```python
from build123d import *

# Parameters (mm, degrees)
BOSS_EXTRUDE1_DEPTH      = 4.5
BOSS_EXTRUDE1_DEPTH_BACK = 4.5
SKETCH1_R                = 11.1125
SKETCH1_R_2              = 4.7625
FILLET1_R                = 1
FILLET2_R                = 1


with BuildPart() as part:
    # Sketch1 → Boss-Extrude1 (new, two sides: drawn at the far end of the back side and taken through both)
    with BuildSketch(Plane(origin=(0, 0, 0), x_dir=(1, 0, 0), z_dir=(0, 1, 0)).offset(-BOSS_EXTRUDE1_DEPTH_BACK)):
        with Locations(Location((0, 0, 0), (0, 0, 270))):
            Circle(SKETCH1_R)
        with Locations(Location((0, 0, 0), (0, 0, 270))):
            Circle(SKETCH1_R_2, mode=Mode.SUBTRACT)
    extrude(amount=BOSS_EXTRUDE1_DEPTH + BOSS_EXTRUDE1_DEPTH_BACK)

    # Fillet1
    fillet1_edges = [part.edges().sort_by_distance(p)[0] for p in [
        (0, -4.5, -4.7625),
        (0, 4.5, -4.7625),
    ]]
    fillet(fillet1_edges, radius=FILLET1_R)

    # Fillet2
    fillet2_edges = [part.edges().sort_by_distance(p)[0] for p in [
        (0, -4.5, -11.1125),
        (0, 4.5, -11.1125),
    ]]
    fillet(fillet2_edges, radius=FILLET2_R)


solid = part.part
```
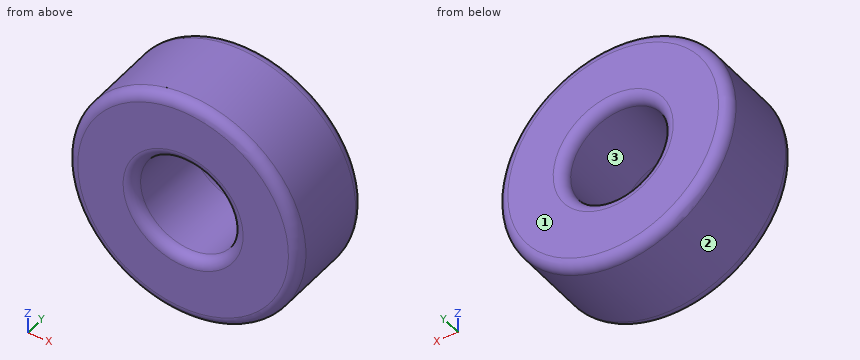
For this review, take the finished solid that the model builds, in its own axes (mm). Face numbers are marked on the shaded views. Give positions to 0.01 mm unless a question says otherwise; leave off trailing zeros. Order: outer loops, then holes, each group sorted by start corner. A loop starts at its lowest first (then second) coordinate and runs counter-clockwise, first axis right, second up.
1) Take a section at B-B (z = 0). Give the boundary of the cut face in (x, y), then the cut area to 3 significant figures.
2) Take a section at A-A (x = 0). Give the boundary of the cut face in (y, z).
3) Take a section at C-C (y = -2.75). Give the boundary of the cut face in (x, z) (1 decimal), then the cut area to 3 significant figures.
4) Wall thickness on line 1 (X direction, y = -2, z = 0); line 2 (X direction, y = -1, z = -2); line 3 (Z direction, x = -3.25, y = -1.5): over which ranges is each line inside the solid? List them lowest first.
5) Insertion check: pin 1 (11 mm diameter, centred on x = 0, z = 0, fed in from +Y); pin 2 (2 mm diameter, centred on x = 8.5, z = -8, fed in from +Y); pin 3 (2 mm diameter, centred on x = -4, y = 3, fed in from +Z). Each pin has a flat end and moves straight along its axis. Give the tip position at first contact, or say it passes through.
6) The part is to be moulded in two halves that separate along X. For the marked faces 1, 2 and 3, say which applies: released by +X, released by -X, zero draft, split by the parting line, or undercut.
Derived:
1. outline: (-11.11, -3.5) arc R1 ccw to (-10.11, -4.5) - (-5.76, -4.5) arc R1 ccw to (-4.76, -3.5) - (-4.76, 3.5) arc R1 ccw to (-5.76, 4.5) - (-10.11, 4.5) arc R1 ccw to (-11.11, 3.5) - close; (4.76, -3.5) arc R1 ccw to (5.76, -4.5) - (10.11, -4.5) arc R1 ccw to (11.11, -3.5) - (11.11, 3.5) arc R1 ccw to (10.11, 4.5) - (5.76, 4.5) arc R1 ccw to (4.76, 3.5) - close
1. area: 113 mm2
2. outline: (-4.5, -10.11) arc R1 ccw to (-3.5, -11.11) - (3.5, -11.11) arc R1 ccw to (4.5, -10.11) - (4.5, -5.76) arc R1 ccw to (3.5, -4.76) - (-3.5, -4.76) arc R1 ccw to (-4.5, -5.76) - close; (-4.5, 5.76) arc R1 ccw to (-3.5, 4.76) - (3.5, 4.76) arc R1 ccw to (4.5, 5.76) - (4.5, 10.11) arc R1 ccw to (3.5, 11.11) - (-3.5, 11.11) arc R1 ccw to (-4.5, 10.11) - close
3. outline: circle Ø22.2 at (0, 0); hole circle Ø9.5 at (0, 0)
3. area: 317 mm2
4. line 1: x = -11.11 to -4.76, 4.76 to 11.11
4. line 2: x = -10.93 to -4.32, 4.32 to 10.93
4. line 3: z = -10.63 to -3.48, 3.48 to 10.63
5. pin 1: stops at y = 4.46
5. pin 2: stops at y = 4.33
5. pin 3: stops at z = 10.7
6. face 1: zero draft
6. face 2: split by the parting line
6. face 3: undercut
